from build123d import *

# Parameters (mm, degrees)
F1_DEPTH = 115
F2_W     = 9
F2_H     = 5
F3_DEPTH = 2
F4_R     = 2


with BuildPart() as f1:
    # F0 (on Top) → F1 (new body)
    with BuildSketch(Plane.XY):
        Polygon((0, 5), (0, 0), (2, 0), (2, 3), (7, 3), (7, 0), (9, 0), (9, 5), align=None)
    extrude(amount=F1_DEPTH)

    # F2 (on Top) → F3 (join)
    with BuildSketch(Plane.XY):
        with Locations((4.5, 2.5)):
            Rectangle(F2_W, F2_H)
    extrude(amount=-F3_DEPTH)

    # F4
    f4_edges = [f1.edges().sort_by_distance(p)[0] for p in [
        (4.5, 5, -2),
        (9, 5, 56.5),
        (9, 2.5, -2),
    ]]
    fillet(f4_edges, radius=F4_R)


solid = f1.part
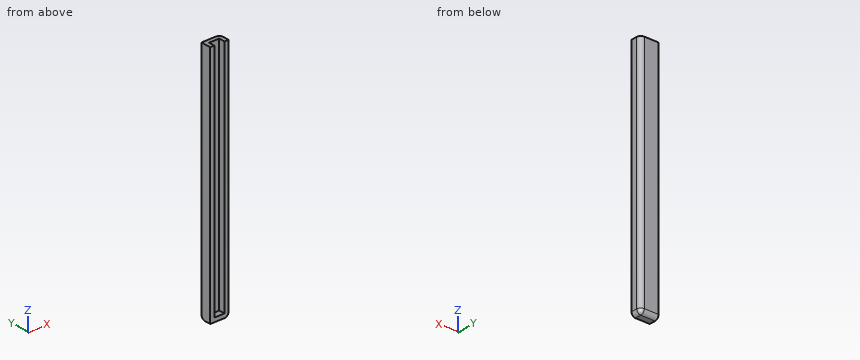
Design review of the part built by this model. Coordinates are the model's own, in mm. Coordinates: 2 decimals unless noted, no trailing zeros. Write each loop counter-clockwise with the first axis right and the second up, starting at its lowest first coordinate (ties: lowest second). Pieces come first, ordered by that corner, then holes. Notation, with made-up numbers: (67.25, 62) - (72.25, 62) arc R26 ccw to (72.25, 86) - close; hole circle Ø3 at (6.25, -26.75). An arc over 180 degrees is marked (long way). One line per item, written item: value.
1) Add section C-C (x = 3.5). State the section outline as (y, z) points, plus the area to 3 significant figures.
Answer sheet:
outline: (0, -2) - (3, -2) arc R2 ccw to (5, 0) - (5, 115) - (3, 115) - (3, 0) - (0, 0) - close
area: 239 mm2
2) Add section D-D (x = 8). State the section outline as (y, z) points, plus the area to 3 significant figures.
Answer sheet:
outline: (0, -1.73) - (3, -1.73) arc R1.73 ccw to (4.73, 0) - (4.73, 115) - (0, 115) - close
area: 552 mm2
3) Add section B-B (y = 1.2). State the section outline as (x, z) points.
Answer sheet:
outline: (0, -2) - (7, -2) arc R2 ccw to (9, 0) - (9, 115) - (7, 115) - (7, 0) - (2, 0) - (2, 115) - (0, 115) - close
4) Insertion check: pin 1 (0.9 mm diameter, centred on x = 4.5, y = 1.5, fed in from +Z); pin 2 (1 mm diameter, centred on x = 3.5, z = 76.5, fed in from -Y). Each pin has a flat end and moves straight along its axis. Give the tip position at first contact, or say it passes through.
Answer sheet:
pin 1: stops at z = 0
pin 2: stops at y = 3
5) Add section A-A (z = 46.5). State the section outline as (x, y) points, plus the area to 3 significant figures.
Answer sheet:
outline: (0, 0) - (2, 0) - (2, 3) - (7, 3) - (7, 0) - (9, 0) - (9, 3) arc R2 ccw to (7, 5) - (0, 5) - close
area: 29.1 mm2
6) To check wall thickness, follow probe 1 along X at (y, z) = (1.1, 3); probe 2 along Y at (x, z) = (4.25, 25.5); probe 3 along X at (y, z) = (3.3, 28.5). State the ranges of each line that lie inside material, in increasing order.
Answer sheet:
probe 1: x = 0 to 2, 7 to 9
probe 2: y = 3 to 5
probe 3: x = 0 to 8.98
